Source: CAD feature listing. Evaluate the final solid. Frame: model axes, mm. Give positions to 0.01 mm unless a question says otherwise; leave off trailing zeros. Order: outer loops, then holes, each group sorted by start corner. A loop starts at its lowest first (then second) coordinate and runs counter-clockwise, first axis right, second up.
```python
from build123d import *

# Parameters (mm, degrees)
SKETCH2_W               = 180
SKETCH2_H               = 9
BOSS_EXTRUDE1_DEPTH     = 14.8
SKETCH7_W               = 90
SKETCH7_H               = 4.5
CUT_EXTRUDE1_DEPTH      = 92.319713096
FILLET1_R               = 8
BOSS_EXTRUDE2_DEPTH     = 14.8
CUT_EXTRUDE2_DEPTH      = 175.130679781
CUT_EXTRUDE2_DEPTH_BACK = 175.130679781
SKETCH11_R              = 2
CUT_EXTRUDE3_DEPTH      = 107.467114171
CUT_EXTRUDE3_DEPTH_BACK = 107.467114171


with BuildPart() as part:
    # Sketch2 → Boss-Extrude1 (new body)
    with BuildSketch(Plane(origin=(0, 0, 0), x_dir=(0, 0, -1), z_dir=(1, 0, 0))):
        Rectangle(SKETCH2_W, SKETCH2_H)
    extrude(amount=BOSS_EXTRUDE1_DEPTH)

    # Sketch7 → Cut-Extrude1 (cut, through all)
    with BuildSketch(Plane(origin=(14.8, 0, 0), x_dir=(0, 0, -1), z_dir=(1, 0, 0))):
        with Locations((0, -2.25)):
            Rectangle(SKETCH7_W, SKETCH7_H)
    extrude(amount=-CUT_EXTRUDE1_DEPTH, mode=Mode.SUBTRACT)

    # Fillet1
    # the kernel refuses this fillet: 8 mm, written as the material it adds along each edge
    with BuildSketch(Plane(origin=(14.8, 0, -45), x_dir=(0, -1, 0), z_dir=(-1, 0, 0))) as fillet1_piece_1:
        with BuildLine():
            CenterArc((8, 7.193747285), FILLET1_R, 180, 64.055520228)
            Line((0, 7.193747285), (-0.16, 7.193747285))
            Line((-0.16, 7.193747285), (-0.16, 0))
            Line((-0.16, 0), (0, -0.16))
            ThreePointArc((0, -0.16), (2.25, -0.16), (4.43, -0.143874946))
            Line((4.43, -0.143874946), (4.5, 0))
        make_face()
    extrude(amount=14.8)
    with BuildSketch(Plane(origin=(14.8, 0, 45), x_dir=(0, -1, 0), z_dir=(-1, 0, 0))) as fillet1_piece_2:
        with BuildLine():
            CenterArc((8, -7.193747285), FILLET1_R, 115.944479772, 64.055520228)
            Line((0, -7.193747285), (-0.16, -7.193747285))
            Line((-0.16, -7.193747285), (-0.16, 0))
            Line((-0.16, 0), (0, 0.16))
            ThreePointArc((0, 0.16), (2.25, 0.16), (4.43, 0.143874946))
            Line((4.43, 0.143874946), (4.5, 0))
        make_face()
    extrude(amount=14.8)

    # Sketch8 → Boss-Extrude2 (add)
    with BuildSketch(Plane(origin=(14.8, 0, 0), x_dir=(0, 0, -1), z_dir=(1, 0, 0))):
        with BuildLine():
            Line((83.579, -39.5), (83.579, -54.92))
            Line((83.579, -54.92), (74.579, -54.92))
            Line((74.579, -54.92), (74.579, -45.7))
            ThreePointArc((74.579, -45.7), (80.779, -39.5), (74.579, -33.3))
            Line((74.579, -33.3), (74.579, -4.5))
            Line((74.579, -4.5), (83.579, -4.5))
            Line((83.579, -4.5), (83.579, -39.5))
        make_face()
        with BuildLine():
            Line((-74.579, -54.92), (-74.579, -45.7))
            ThreePointArc((-74.579, -45.7), (-80.779, -39.5), (-74.579, -33.3))
            Line((-74.579, -33.3), (-74.579, -4.5))
            Line((-74.579, -4.5), (-83.579, -4.5))
            Line((-83.579, -4.5), (-83.579, -39.5))
            Line((-83.579, -39.5), (-83.579, -54.92))
            Line((-83.579, -54.92), (-74.579, -54.92))
        make_face()
    extrude(amount=-BOSS_EXTRUDE2_DEPTH)

    # Sketch11 → Cut-Extrude2 (cut, two sides: drawn at the far end of the back side and taken through both)
    with BuildSketch(Plane(origin=(0, 0, 74.579), x_dir=(-1, 0, 0), z_dir=(0, 0, -1)).offset(-CUT_EXTRUDE2_DEPTH_BACK)):
        with Locations(Location((-7.4, -28.8, 0), (0, 0, 180))):
            Circle(SKETCH11_R)
        with Locations(Location((-7.4, -50.2, 0), (0, 0, 180))):
            Circle(SKETCH11_R)
    extrude(amount=CUT_EXTRUDE2_DEPTH + CUT_EXTRUDE2_DEPTH_BACK, mode=Mode.SUBTRACT)

    # Sketch12 → Cut-Extrude3 (cut, two sides: drawn at the far end of the back side and taken through both)
    with BuildSketch(Plane.ZY.offset(-CUT_EXTRUDE3_DEPTH_BACK)):
        Polygon((96.986162818, 8.741450318), (-95.153164269, 8.741450318), (-95.153164269, -16.038890922), (-95.153164269, -24.08), (-95.153164269, -55.626735024), (-68.956122855, -55.626735024), (-68.956122855, -24.08), (74.579, -24.08), (96.986162818, -24.08), (96.986162818, -16.038890922), (96.986162818, -4.5), align=None)
    extrude(amount=CUT_EXTRUDE3_DEPTH + CUT_EXTRUDE3_DEPTH_BACK, mode=Mode.SUBTRACT)


solid = part.part
```
1) Section query C-C, the plane x = 7.4. Return the cut outline in (y, z), and give its area (3 significant figures).
Report:
outline: (-54.92, 74.58) - (-52.2, 74.58) - (-52.2, 83.58) - (-54.92, 83.58) - close; (-48.2, 74.58) - (-45.7, 74.58) arc R6.2 cw to (-33.3, 74.58) - (-30.8, 74.58) - (-30.8, 83.58) - (-48.2, 83.58) - close; (-26.8, 74.58) - (-24.08, 74.58) - (-24.08, 83.58) - (-26.8, 83.58) - close
area: 145 mm2
2) Material intervals for L1, parallel to Y at x = 6.25, z = 76.75; L2, parallel to Y at x = 7.4, z = 81.5; L3, parallel to Y at x = 7.4, z = 79.75, sorted ascending.
Report:
L1: y = -54.92 to -51.84, -48.56 to -45.31, -33.69 to -30.44, -27.16 to -24.08
L2: y = -54.92 to -52.2, -48.2 to -30.8, -26.8 to -24.08
L3: y = -54.92 to -52.2, -48.2 to -42.92, -36.08 to -30.8, -26.8 to -24.08
3) Section query B-B, the plane y = -28.8. Return the cut outline in (x, z), and give its area (3 significant figures).
Report:
outline: (0, 74.58) - (5.4, 74.58) - (5.4, 83.58) - (0, 83.58) - close; (9.4, 74.58) - (14.8, 74.58) - (14.8, 83.58) - (9.4, 83.58) - close
area: 97.2 mm2
4) Section query D-D, the plane z = 83.25. Return the cut outline in (x, y).
Report:
outline: (0, -54.92) - (14.8, -54.92) - (14.8, -24.08) - (0, -24.08) - close; hole circle Ø4 at (7.4, -50.2); hole circle Ø4 at (7.4, -28.8)
5) Draft query along Y for faces 1 (the cylindrical face through (7.504, -39.636, 80.778)), 2 (the cylindrical face through (8.323, -48.426, 79.142)), 3 (the flat face through (7.5, -52.4, 74.579)), 4 (the flat face through (8, -24.08, 79)). Return one class per face: +Y half, -Y half, draft (parallel to the pull), parting line (faces both ways), or undercut.
Report:
face 1: undercut
face 2: undercut
face 3: draft
face 4: +Y half
6) Section query A-A, the plane z = 79.25. Return the cut outline in (x, y), and give its area (3 significant figures).
Report:
outline: (0, -54.92) - (14.8, -54.92) - (14.8, -43.58) - (0, -43.58) - close; (0, -35.42) - (14.8, -35.42) - (14.8, -24.08) - (0, -24.08) - close; hole circle Ø4 at (7.4, -50.2); hole circle Ø4 at (7.4, -28.8)
area: 311 mm2
